```python
from build123d import *

# Parameters (mm, degrees)
SKETCH1_R           = 10.000000000000009
BOSS_EXTRUDE1_DEPTH = 23
FILLET1_R           = 20
FILLET2_R           = 8


with BuildPart() as part:
    # Sketch1 → Boss-Extrude1 (new body)
    # profile 1 of 8: a face of its own
    with BuildSketch(Plane(origin=(0, 0, 0), x_dir=(1, 0, 0), z_dir=(0, 1, 0))):
        with BuildLine():
            Line((190.53750510204208, 11.499999999999996), (-169.0643228571688, 11.499999999999996))
            ThreePointArc((-169.06432285716886, 11.499999999999785), (-167.29719813473903, 5.8702645292353655), (-166.699999999998, -5.84695e-12))
            ThreePointArc((-166.699999999998, -5.85409e-12), (-167.29719813473773, -5.870264529240628), (-169.0643228571637, -11.499999999999407))
            Line((-169.0643228571635, -11.499999999999996), (190.53750510204208, -11.499999999999996))
            ThreePointArc((190.53750510204202, -11.500000000000126), (186.70000000000027, 2.35e-15), (190.53750510204205, 11.500000000000131))
        make_face()
    # profile 2 of 8: a face of its own
    with BuildSketch(Plane(origin=(0, 0, 0), x_dir=(1, 0, 0), z_dir=(0, 1, 0))):
        with BuildLine():
            Line((-209.0364197819809, 13.186419781973054), (-191.02343537482668, 18.01298440714431))
            Line((-191.02343537482668, 18.01298440714431), (-184.51045096768246, 11.499999999999996))
            Line((-184.51045096768246, 11.499999999999996), (-169.0643228571688, 11.499999999999996))
            ThreePointArc((-169.06432285716886, 11.499999999999785), (-195.8499999999993, 29.149999999995877), (-222.63567714283025, 11.500000000000531))
            Line((-222.63567714283008, 11.499999999999996), (-215.33022409119366, 11.499999999999996))
            Line((-215.33022409119366, 11.500000000000018), (-209.0364197819809, 13.186419781973054))
        make_face()
    # profile 3 of 8: a face of its own
    with BuildSketch(Plane(origin=(0, 0, 0), x_dir=(1, 0, 0), z_dir=(0, 1, 0))):
        with BuildLine():
            Line((-169.0643228571688, 11.499999999999996), (-184.51045096768246, 11.499999999999996))
            Line((-184.51045096768246, 11.499999999999996), (-177.83701559284398, 4.826564625161424))
            Line((-177.83701559284398, 4.826564625161426), (-182.21170539933064, -11.499999999999996))
            Line((-182.21170539933064, -11.499999999999996), (-169.0643228571635, -11.499999999999996))
            ThreePointArc((-169.0643228571637, -11.499999999999407), (-167.29719813473773, -5.870264529240628), (-166.699999999998, -5.85409e-12))
            ThreePointArc((-166.699999999998, -5.84695e-12), (-167.29719813473903, 5.8702645292353655), (-169.06432285716886, 11.499999999999785))
        make_face()
    # profile 4 of 8: a face of its own
    with BuildSketch(Plane(origin=(0, 0, 0), x_dir=(1, 0, 0), z_dir=(0, 1, 0))):
        with BuildLine():
            Line((-169.0643228571635, -11.499999999999996), (-182.21170539933064, -11.499999999999996))
            Line((-182.21170539933064, -11.499999999999996), (-182.66358021801545, -13.186419781992653))
            Line((-182.66358021801545, -13.186419781992653), (-200.67656462516962, -18.012984407163884))
            Line((-200.67656462516962, -18.012984407163888), (-215.11044742166933, -21.880531646131363))
            ThreePointArc((-215.11044742167047, -21.88053164613265), (-189.43937367309758, -28.43635648421335), (-169.0643228571637, -11.499999999999407))
        make_face()
    # profile 5 of 8: a face of its own
    with BuildSketch(Plane(origin=(0, 0, 0), x_dir=(1, 0, 0), z_dir=(0, 1, 0))):
        with BuildLine():
            Line((221.162494897959, 11.499999999999996), (190.53750510204208, 11.499999999999996))
            ThreePointArc((190.53750510204205, 11.500000000000131), (186.70000000000027, 2.35e-15), (190.53750510204202, -11.500000000000126))
            Line((190.53750510204208, -11.499999999999996), (221.162494897959, -11.499999999999996))
            ThreePointArc((221.16249489795885, -11.499999999999684), (224.0153072819582, -6.061692119536153), (225.00000000000028, -4.69e-15))
            ThreePointArc((225.00000000000028, 0), (224.0153072819582, 6.061692119536143), (221.16249489795888, 11.49999999999967))
        make_face()
        with Locations(Location((205.85000000000028, 0, 0), (0, 0, 270))):
            Circle(SKETCH1_R, mode=Mode.SUBTRACT)
    # profile 6 of 8: a face of its own
    with BuildSketch(Plane(origin=(0, 0, 0), x_dir=(1, 0, 0), z_dir=(0, 1, 0))):
        with BuildLine():
            Line((221.162494897959, -11.499999999999996), (190.53750510204208, -11.499999999999996))
            ThreePointArc((190.53750510204202, -11.500000000000126), (205.85000000000053, -19.150000000000006), (221.16249489795885, -11.499999999999684))
        make_face()
    # profile 7 of 8: a face of its own
    with BuildSketch(Plane(origin=(0, 0, 0), x_dir=(1, 0, 0), z_dir=(0, 1, 0))):
        with BuildLine():
            ThreePointArc((221.16249489795888, 11.49999999999967), (205.85000000000056, 19.150000000000006), (190.53750510204205, 11.500000000000131))
            Line((190.53750510204208, 11.499999999999996), (221.162494897959, 11.499999999999996))
        make_face()
    # profile 8 of 8: a face of its own
    with BuildSketch(Plane(origin=(0, 0, 0), x_dir=(1, 0, 0), z_dir=(0, 1, 0))):
        with BuildLine():
            Line((-223.47030257848598, 9.31887254300414), (-215.33022409119366, 11.500000000000018))
            Line((-215.33022409119366, 11.499999999999996), (-222.63567714283008, 11.499999999999996))
            ThreePointArc((-222.63567714283025, 11.500000000000519), (-223.0748413513289, 10.417797914863556), (-223.4703025784876, 9.318872543004696))
        make_face()
    extrude(amount=BOSS_EXTRUDE1_DEPTH)

    # Fillet1
    fillet1_edges = [part.edges().sort_by_distance(p)[0] for p in [
        (-169.06432285716357, 11.5, 11.499999999999702),
        (-169.06432285716883, 11.5, -11.499999999999892),
        (190.53750510204208, 11.5, -11.500000000000068),
        (190.53750510204205, 11.5, 11.500000000000059),
    ]]
    fillet(fillet1_edges, radius=FILLET1_R)

    # Fillet2
    fillet2_edges = [part.edges().sort_by_distance(p)[0] for p in [
        (-193.61734753029688, 0, 29.06437274310201),
        (225.00000000000028, 0, -2.576e-14),
        (225.0000000000003, 23, -4.174e-14),
        (12.240435042127586, 0, 11.499999999999766),
        (12.240435042127586, 23, 11.499999999999766),
        (12.24043504212267, 0, -11.499999999999865),
        (12.240435042122641, 23, -11.499999999999865),
        (-201.21583651826683, 0, -28.651881237695218),
        (-201.21583651826677, 23, -28.651881237695314),
        (188.85337218093906, 0, 12.50211748036416),
        (-193.61734753029688, 23, 29.06437274310201),
        (188.85337218093903, 23, 12.502117480364152),
        (188.85337218093898, 0, -12.502117480364163),
        (188.85337218093898, 23, -12.502117480364163),
        (-166.59579003361372, 0, -13.384287379634728),
        (-166.59579003361372, 23, -13.384287379634728),
        (-166.5957900336068, 0, 13.384287379636046),
        (-166.5957900336068, 23, 13.384287379636042),
    ]]
    fillet(fillet2_edges, radius=FILLET2_R)


solid = part.part
```
Can you work these out from the model? Positions are in its coordinate system, mm. A direction names the side the tool comes from. Round coordinates to 2 decimals unless told otherwise and drop trailing zeros. Order: outer loops, then holes, each group sorted by start corner. A loop starts at its lowest first (then second) coordinate and runs counter-clockwise, first axis right, second up. Notation, with made-up numbers: (44, 69.5) -> (70, 69.5) arc R25 cw to (70, 93.5) -> close; hole circle Ø8 at (53.25, 87.25). An arc over 180 degrees is marked (long way). Return JSON: item names as keys, results as strings. Group by question number.
1. Will these pins go through, and if not, where does the flat tip stop? pin 1 (7.5 mm diameter, centred on x = 16.5, y = 13, fed in from +Z); pin 2 (2 mm diameter, centred on x = 62.5, y = 11.5, fed in from -Z); pin 3 (5 mm diameter, centred on x = -118.5, z = -9.5, fed in from +Y).
2. If we section it at A-A, the plane x = -133: Write out the boundary of the cut face in (y, z), then the cut area to 3 significant figures.
3. We'd pull the mould along X, two halves only. Please class faces 1 (the face through (-198.66, 11.339, 17.473)), 2 (the face through (-15, 0, 0)), 3 (the face through (10, 11, 11.5)), 4 (the face through (14.625, 2.281, 9.094)): released by +X, released by -X, zero draft, split by the parting line, or undercut.
4. I need wall thicknesses on line 1 (Z direction, x = -86, y = 15.5); line 2 (X direction, y = 6.25, z = 0); line 3 (X direction, y = 4.75, z = 0). Which ranges of each line are inside material? Lowest first, please. Write a range as [from, to].
5. Which directions (+Z, -Z, +X, -X, +Y, -Y) give clear straight access to the entire face, cutting with the end or side of a thin tool? Please do faces 5 (the face through (-166.48, 11.55, 13.33)), 6 (the face through (188.769, 11.549, -12.474)), 7 (the face through (-207.5, 11.3, -13.6)), 8 (the face through (9.855, 2.281, -9.094)).
Output values:
{
 "1": {"pin 1": "z = 11.5", "pin 2": "z = -11.5", "pin 3": "y = 22.19"},
 "2": {"outline": "(0, -3.5) arc R8 ccw to (8, -11.5) -> (15, -11.5) arc R8 ccw to (23, -3.5) -> (23, 3.5) arc R8 ccw to (15, 11.5) -> (8, 11.5) arc R8 ccw to (0, 3.5) -> close", "area": "474 mm²"},
 "3": {"face 1": "released by -X", "face 2": "zero draft", "face 3": "undercut", "face 4": "undercut"},
 "4": {"line 1": "[-11.48, 11.48]", "line 2": "[-179.13, 195.85], [215.85, 224.81]", "line 3": "[-179.13, 195.85], [215.85, 224.31]"},
 "5": {"face 5": "+Z, +Y, -Y", "face 6": "-Z, +Y, -Y", "face 7": "+Y, -Y", "face 8": "-Z, -Y"}
}
